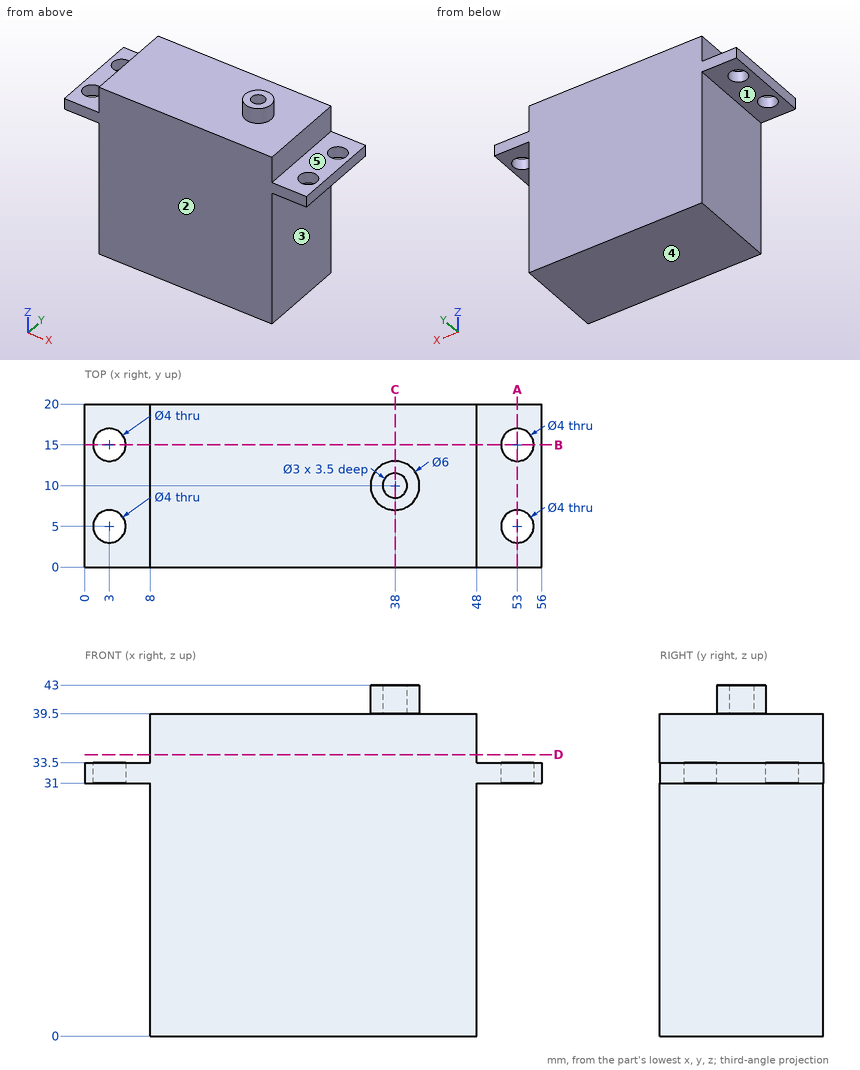
Here's the drawing with two shaded views (mm, measured from the low corner). I have some questions. A direction names the side the tool comes from. Give positions to 0.01 mm unless a question says otherwise; leave off trailing zeros. Order: outer loops, then holes, each group sorted by start corner. A loop starts at its lowest first (then second) coordinate and runs counter-clockwise, first axis right, second up. Notation, with made-up numbers: (51.25, 2) -> (61.25, 2) arc R20 ccw to (61.25, 17) -> close; hole circle Ø5 at (89, -9). An arc over 180 degrees is marked (long way). One line per item, written item: value. Start each with the question number.
1. Will these pins go through, and if not, where does the flat tip stop? pin 1 Ø4 at (x, z) = (21, 12) entering from -Y; pin 2 Ø9 at (x, y) = (50.5, 14) entering from +Z; pin 3 Ø4.5 at (x, y) = (3, 5) entering from -Z; pin 4 Ø10 at (y, z) = (2, 10.5) entering from -X.
2. Imagine slicing it at D-D, the plane z = 34.5. List the corners of the cut face in (x, y) for me, plus the area to 3 significant figures.
3. Imagine slicing it at A-A, the plane x = 53. List the corners of the cut face in (y, z) for me.
4. For the marked faces 1, 2, 3, 4 and 5, which set-ups out of +Z, -Z, +X, -X, +Y, -Y let a thin tool reach every point of the face, with its end or its side?
5. Imagine slicing it at C-C, the plane x = 38. List the corners of the cut face in (y, z) for me, plus the area to 4 significant figures.
6. I need wall thicknesses on probe 1 along Y at (x, z) = (53, 32); probe 2 along X at (y, z) = (6, 38.5); probe 3 along Z at (x, y) = (20, 6.25). Which ranges of each line are inside material? Lowest first, please. Write a range as from..to.
7. Imagine slicing it at B-B, the plane y = 15. List the corners of the cut face in (x, z) for me.
Values follow:
1. pin 1: stops at y = 0
1. pin 2: stops at z = 39.5
1. pin 3: stops at z = 31
1. pin 4: stops at x = 8
2. outline: (8, 0) -> (48, 0) -> (48, 20) -> (8, 20) -> close
2. area: 800 mm2
3. outline: (0, 31) -> (3, 31) -> (3, 33.5) -> (0, 33.5) -> close; (7, 31) -> (13, 31) -> (13, 33.5) -> (7, 33.5) -> close; (17, 31) -> (20, 31) -> (20, 33.5) -> (17, 33.5) -> close
4. face 1: -Z, -X, +Y, -Y
4. face 2: +Z, -Z, +X, -X, -Y
4. face 3: -Z, +X, +Y, -Y
4. face 4: -Z, +X, -X, +Y, -Y
4. face 5: +Z, +X, +Y, -Y
5. outline: (0, 0) -> (20, 0) -> (20, 39.5) -> (13, 39.5) -> (13, 43) -> (11.5, 43) -> (11.5, 39.5) -> (8.5, 39.5) -> (8.5, 43) -> (7, 43) -> (7, 39.5) -> (0, 39.5) -> close
5. area: 800.5 mm2
6. probe 1: y = 0..3, 7..13, 17..20
6. probe 2: x = 8..48
6. probe 3: z = 0..39.5
7. outline: (0, 31) -> (1, 31) -> (1, 33.5) -> (0, 33.5) -> close; (5, 31) -> (8, 31) -> (8, 0) -> (48, 0) -> (48, 31) -> (51, 31) -> (51, 33.5) -> (48, 33.5) -> (48, 39.5) -> (8, 39.5) -> (8, 33.5) -> (5, 33.5) -> close; (55, 31) -> (56, 31) -> (56, 33.5) -> (55, 33.5) -> close
